Autodesk Inventor part; units mm, degrees
ref_plane "YZ Plane" through (0, 0, 0) normal (1, 0, 0) x (0, 1, 0)
ref_plane "XZ Plane" through (0, 0, 0) normal (0, 1, 0) x (-1, 0, 0)
ref_plane "XY Plane" through (0, 0, 0) normal (0, 0, 1) x (1, 0, 0)
sketch "Sketch1" plane through (0, 0, 0) normal (0, 1, 0) x (-1, 0, 0)
  line L0 (-125, 125) -> (125, 125)
  line L1 (125, 125) -> (125, -125)
  line L2 (125, -125) -> (-125, -125)
  line L3 (-125, -125) -> (-125, 125)
  line L4 (-125, 125) -> (125, -125) construction
  line L5 (125, 125) -> (-125, -125) construction
  point P0 (0, 0)
  dimension "d0" = 250
extrude "Extrusion1" add sketch "Sketch1" along normal mid plane 60
sketch "Sketch2" plane through (0, 30, 0) normal (0, 1, 0) x (1, 0, 0)
  line L0 (-100, -100) -> (100, -100)
  line L1 (100, -100) -> (100, 100)
  line L2 (100, 100) -> (-100, 100)
  line L3 (-100, 100) -> (-100, -100)
  line L4 (-100, -100) -> (100, 100) construction
  line L5 (100, -100) -> (-100, 100) construction
  point P0 (0, 0)
  dimension "d3" = 200
extrude "Extrusion2" cut sketch "Sketch2" against normal blind 50.4
properties part number "Box"
Read the model definition and answer for the solid it produces. Units are mm, in the model's axes. A direction names the side the tool comes from. Coordinates: 2 decimals unless noted, no trailing zeros. Write each loop counter-clockwise with the first axis right and the second up, starting at its lowest first coordinate (ties: lowest second). Pieces come first, ordered by that corner, then holes. Notation, with made-up numbers: (46, 7) - (54, 7) arc R35 cw to (54, 46) - close; hole circle Ø8 at (58, -18). An arc over 180 degrees is marked (long way). One line per question, with ' | ' between items.
Q1. Consider L1, parallel to Z at x = 15, y = -2.5; L2, parallel to Y at x = 68, z = 18. Determine where each line is inside the solid, lowest interval first. Write a range as [from, to].
Result set:
L1: [-125, -100], [100, 125] | L2: [-30, -20.4]
Q2. Find section A-A, the plane x = -84.5. Write down the section's boundary in (y, z), plus the area to 3 significant figures.
Result set:
outline: (-30, -125) - (30, -125) - (30, -100) - (-20.4, -100) - (-20.4, 100) - (30, 100) - (30, 125) - (-30, 125) - close | area: 4,920 mm^2
Q3. Find section C-C, the plane z = 25. Write down the section's boundary in (x, y), plus the area to 3 significant figures.
Result set:
outline: (-125, -30) - (125, -30) - (125, 30) - (100, 30) - (100, -20.4) - (-100, -20.4) - (-100, 30) - (-125, 30) - close | area: 4,920 mm^2
Q4. Find section B-B, the plane y = 25. Write down the section's boundary in (x, z).
Result set:
outline: (-125, -125) - (125, -125) - (125, 125) - (-125, 125) - close; hole (-100, -100) - (100, -100) - (100, 100) - (-100, 100) - close
Q5. For faces 4 (the flat face through (-125, 0, 2)), 5 (the flat face through (-1, 5, 100)), determine the directions among +Z, -Z, +X, -X, +Y, -Y from which every point of the face is accessible in a straight line to the end or side of a thin tool.
Result set:
face 4: +Z, -Z, -X, +Y, -Y | face 5: +Y
Q6. This flat-tipped pin is pushed along its axis until it touches: P1, Ø5, axis at x = 95, z = -25.5, coming from the +Y side. Where does it stop, or does it pass through?
Result set:
P1: y = -20.4
Q7. Determine the mould class of faces 1 (the flat face through (-2, 0, -125)), 2 (the flat face through (113, 30, 2)), 3 (the flat face through (100, 5, 1)) for opening direction Z: +Z half, -Z half, draft (parallel to the pull), parting line (faces both ways), or undercut.
Result set:
face 1: -Z half | face 2: draft | face 3: undercut
